```python
from build123d import *

# Parameters (mm, degrees)
SKETCH1_W           = 482.6
SKETCH1_H           = 101.6
BOSS_EXTRUDE1_DEPTH = 12.7
SKETCH2_R           = 2.7813
CUT_EXTRUDE1_DEPTH  = 13.7
SKETCH3_R           = 1.5875
CUT_EXTRUDE2_DEPTH  = 13.7
SKETCH4_R           = 0.79375
CUT_EXTRUDE3_DEPTH  = 13.7
SKETCH5_R           = 0.79375
CUT_EXTRUDE4_DEPTH  = 13.7
CUT_EXTRUDE5_DEPTH  = 13.7


with BuildPart() as part:
    # Sketch1 → Boss-Extrude1 (new body)
    with BuildSketch(Plane(origin=(0, 0, 0), x_dir=(1, 0, 0), z_dir=(0, 1, 0))):
        Rectangle(SKETCH1_W, SKETCH1_H)
    extrude(amount=BOSS_EXTRUDE1_DEPTH)

    # Sketch2 → Cut-Extrude1 (cut, through all)
    with BuildSketch(Plane(origin=(0, 12.7, 0), x_dir=(1, 0, 0), z_dir=(0, 1, 0))):
        with Locations((-232.5624, 38.1)):
            Circle(SKETCH2_R)
        with Locations((-232.5624, -38.1)):
            Circle(SKETCH2_R)
        with Locations((232.5624, 38.1)):
            Circle(SKETCH2_R)
        with Locations((232.5624, -38.1)):
            Circle(SKETCH2_R)
    extrude(amount=-CUT_EXTRUDE1_DEPTH, mode=Mode.SUBTRACT)

    # Sketch3 → Cut-Extrude2 (cut, through all)
    with BuildSketch(Plane(origin=(0, 12.7, 0), x_dir=(1, 0, 0), z_dir=(0, 1, 0))):
        with Locations((-25.4, 25.4)):
            Circle(SKETCH3_R)
        with Locations((25.4, 25.4)):
            Circle(SKETCH3_R)
        with Locations((25.4, -25.4)):
            Circle(SKETCH3_R)
        with Locations((-25.4, -25.4)):
            Circle(SKETCH3_R)
    extrude(amount=-CUT_EXTRUDE2_DEPTH, mode=Mode.SUBTRACT)

    # Sketch4 → Cut-Extrude3 (cut, through all)
    with BuildSketch(Plane(origin=(0, 12.7, 0), x_dir=(1, 0, 0), z_dir=(0, 1, 0))):
        with Locations((-69.85, 12.7)):
            Circle(SKETCH4_R)
        with Locations((-69.85, -12.7)):
            Circle(SKETCH4_R)
        with Locations((69.85, -12.7)):
            Circle(SKETCH4_R)
        with Locations((69.85, 12.7)):
            Circle(SKETCH4_R)
    extrude(amount=-CUT_EXTRUDE3_DEPTH, mode=Mode.SUBTRACT)

    # Sketch5 → Cut-Extrude4 (cut, through all)
    with BuildSketch(Plane(origin=(0, 12.7, 0), x_dir=(1, 0, 0), z_dir=(0, 1, 0))):
        with Locations((127, 0)):
            Circle(SKETCH5_R)
        with Locations((152.4, 0)):
            Circle(SKETCH5_R)
    extrude(amount=-CUT_EXTRUDE4_DEPTH, mode=Mode.SUBTRACT)

    # Sketch6 → Cut-Extrude5 (cut, through all)
    with BuildSketch(Plane(origin=(0, 12.7, 0), x_dir=(1, 0, 0), z_dir=(0, 1, 0))):
        with BuildLine():
            Line((85.725, 7.9375), (85.725, -7.9375))
            ThreePointArc((85.725, -7.9375), (88.9, -11.1125), (92.075, -7.9375))
            Line((92.075, -7.9375), (92.075, 7.9375))
            ThreePointArc((92.075, 7.9375), (88.9, 11.1125), (85.725, 7.9375))
        make_face()
    extrude(amount=-CUT_EXTRUDE5_DEPTH, mode=Mode.SUBTRACT)


solid = part.part
```
Part model, mm, in its own coordinate system. A direction names the side the tool comes from. Give positions to 0.01 mm unless a question says otherwise; leave off trailing zeros. Use a Markdown table: item, result. Add a question column.
(1) Mould opens along X. For faces 1 (the face through (-3, 12.7, -1)), 2 (the face through (241.3, 6, 1)), 3 (the face through (85.725, 6, 0)) say: +X half, -X half, draft (parallel to the pull), parting line (faces both ways), or undercut.
(2) Drop a flat-ended pin along its axis: P1, Ø1, axis at x = 192.5, z = 6, coming from the -Y side. Give the stop position or say it passes through.
(3) 3-axis set-ups, long thin cutter, end or side, ignore diameter. For faces 4 (the face through (92.075, 6, 0)), 5 (the face through (-241.3, 6, 1)): which of +Z, -Z, +X, -X, +Y, -Y reach the whole face in a straight line?
(4) Probe line 1 along Z through (x, y) = (69.85, 6.5); line 2 along X through (y, z) = (7, 38.1); line 3 along X through (y, z) = (8, -25.4). List the from-to ranges inside material, lowest first. Write a range as [from, to].
Answer key:
| question | item | result |
|---|---|---|
| 1 | face 1 | draft |
| 1 | face 2 | +X half |
| 1 | face 3 | undercut |
| 2 | P1 | y = 0 |
| 3 | face 4 | +Y, -Y |
| 3 | face 5 | +Z, -Z, -X, +Y, -Y |
| 4 | line 1 | [-50.8, -13.49], [-11.91, 11.91], [13.49, 50.8] |
| 4 | line 2 | [-241.3, -235.34], [-229.78, 229.78], [235.34, 241.3] |
| 4 | line 3 | [-241.3, -26.99], [-23.81, 23.81], [26.99, 241.3] |
